Geometry: final body of the model. Coordinates: model frame, mm. A direction names the side the tool comes from. Round coordinates to 2 decimals unless told otherwise and drop trailing zeros. Loops run counter-clockwise (first coordinate to the right, second up) from the corner with the lowest first, then second, coordinate; pieces in that order, holes last. Notation, with made-up numbers: (83.5, 23.25) -> (124.5, 23.25) arc R9 cw to (124.5, 33.25) -> close; hole circle Ø10 at (44, 23). An arc over 180 degrees is marked (long way). Answer in a Markdown table with one row per item.
```python
from build123d import *

# Parameters (mm, degrees)
IZIM1_W                     = 170
IZIM1_H                     = 8
Y_KSEKLIK_EKSTR_ZYON1_DEPTH = 60
IZIM2_R                     = 1.6
IZIM2_R_2                   = 2.1
KES_EKSTR_ZYON1_DEPTH       = 5
IZIM3_R                     = 3.4
KES_EKSTR_ZYON2_DEPTH       = 2.7
IZIM4_R                     = 4.4
KES_EKSTR_ZYON3_DEPTH       = 3.5
RADYUS1_R                   = 4
KES_EKSTR_ZYON4_DEPTH       = 10


with BuildPart() as part:
    # Çizim1 → Yükseklik-Ekstrüzyon1 (new, symmetric)
    with BuildSketch(Plane.XY):
        Rectangle(IZIM1_W, IZIM1_H)
    extrude(amount=Y_KSEKLIK_EKSTR_ZYON1_DEPTH, both=True)

    # Çizim2 → Kes-Ekstrüzyon1 (cut, symmetric)
    with BuildSketch(Plane(origin=(0, 0, 0), x_dir=(1, 0, 0), z_dir=(0, 1, 0))):
        with Locations(Location((0, 56, 0), (0, 0, 270))):
            Circle(IZIM2_R)
        with Locations(Location((0, -56, 0), (0, 0, 270))):
            Circle(IZIM2_R)
        with Locations(Location((-76, 0, 0), (0, 0, 270))):
            Circle(IZIM2_R_2)
        with Locations(Location((76, 0, 0), (0, 0, 270))):
            Circle(IZIM2_R_2)
    extrude(amount=KES_EKSTR_ZYON1_DEPTH, both=True, mode=Mode.SUBTRACT)

    # Çizim3 → Kes-Ekstrüzyon2 (cut)
    with BuildSketch(Plane.XZ.offset(4)):
        with Locations(Location((0, -56, 0), (0, 0, 270))):
            Circle(IZIM3_R)
        with Locations(Location((0, 56, 0), (0, 0, 270))):
            Circle(IZIM3_R)
    extrude(amount=-KES_EKSTR_ZYON2_DEPTH, mode=Mode.SUBTRACT)

    # Çizim4 → Kes-Ekstrüzyon3 (cut)
    with BuildSketch(Plane.XZ.offset(4)):
        with Locations(Location((-76, 0, 0), (0, 0, 270))):
            Circle(IZIM4_R)
        with Locations(Location((76, 0, 0), (0, 0, 270))):
            Circle(IZIM4_R)
    extrude(amount=-KES_EKSTR_ZYON3_DEPTH, mode=Mode.SUBTRACT)

    # Radyus1
    # the kernel refuses this fillet: 4 mm, written as the material it takes off along each edge
    with BuildSketch(Plane(origin=(-95, -4, 60), x_dir=(0, 0, -1), z_dir=(1, 0, 0))) as radyus1_piece_1:
        with BuildLine():
            CenterArc((RADYUS1_R, RADYUS1_R), RADYUS1_R, 180, 90)
            Line((0, RADYUS1_R), (0, 0))
            Line((0, 0), (RADYUS1_R, 0))
        make_face()
    extrude(amount=190, mode=Mode.SUBTRACT)
    with BuildSketch(Plane(origin=(-95, -4, -60), x_dir=(0, 0, 1), z_dir=(1, 0, 0))) as radyus1_piece_2:
        with BuildLine():
            CenterArc((RADYUS1_R, -RADYUS1_R), RADYUS1_R, 90, 90)
            Line((0, -RADYUS1_R), (0, 0))
            Line((0, 0), (RADYUS1_R, 0))
        make_face()
    extrude(amount=190, mode=Mode.SUBTRACT)

    # Çizim6 → Kes-Ekstrüzyon4 (cut, symmetric)
    with BuildSketch(Plane(origin=(0, 0, 0), x_dir=(1, 0, 0), z_dir=(0, 1, 0))):
        with BuildLine():
            Line((4.5, -43.24922609), (58.973465944, -43.24922609))
            ThreePointArc((58.973465944, -43.24922609), (59.680572726, -43.542119309), (59.973465944, -44.24922609))
            Line((59.973465944, -44.24922609), (59.973465944, -45.74922609))
            ThreePointArc((59.973465944, -45.74922609), (59.680572726, -46.456332871), (58.973465944, -46.74922609))
            Line((58.973465944, -46.74922609), (-59.026534056, -46.74922609))
            ThreePointArc((-59.026534056, -46.74922609), (-59.733640837, -46.456332871), (-60.026534056, -45.74922609))
            Line((-60.026534056, -45.74922609), (-60.026534056, -44.24922609))
            ThreePointArc((-60.026534056, -44.24922609), (-59.733640837, -43.542119309), (-59.026534056, -43.24922609))
            Line((-59.026534056, -43.24922609), (-4.5, -43.24922609))
            Line((-4.5, -43.24922609), (4.5, -43.24922609))
        make_face()
        with BuildLine():
            Line((-59.026534056, -1.74922609), (-4.5, -1.74922609))
            Line((-4.5, -1.74922609), (4.5, -1.74922609))
            Line((4.5, -1.74922609), (58.973465944, -1.74922609))
            ThreePointArc((58.973465944, -1.74922609), (59.680572726, -1.456332871), (59.973465944, -0.74922609))
            Line((59.973465944, -0.74922609), (59.973465944, 0.747733475))
            ThreePointArc((59.973465944, 0.747733475), (59.68059176, 1.454821222), (58.973519783, 1.747733474))
            Line((58.973519783, 1.747733474), (4.499892323, 1.750666239))
            Line((4.499892323, 1.750666239), (-4.5, 1.75077391))
            Line((-4.5, 1.75077391), (-59.026534056, 1.75077391))
            ThreePointArc((-59.026534056, 1.75077391), (-59.733640837, 1.457880691), (-60.026534056, 0.75077391))
            Line((-60.026534056, 0.75077391), (-60.026534056, -0.74922609))
            ThreePointArc((-60.026534056, -0.74922609), (-59.733640837, -1.456332871), (-59.026534056, -1.74922609))
        make_face()
        with BuildLine():
            Line((4.5, -28.24922609), (58.973465944, -28.24922609))
            ThreePointArc((58.973465944, -28.24922609), (59.680572726, -28.542119309), (59.973465944, -29.24922609))
            Line((59.973465944, -29.24922609), (59.973465944, -30.74922609))
            ThreePointArc((59.973465944, -30.74922609), (59.680572726, -31.456332871), (58.973465944, -31.74922609))
            Line((58.973465944, -31.74922609), (4.5, -31.74922609))
            Line((4.5, -31.74922609), (-4.5, -31.74922609))
            Line((-4.5, -31.74922609), (-59.026534056, -31.74922609))
            ThreePointArc((-59.026534056, -31.74922609), (-59.733640837, -31.456332871), (-60.026534056, -30.74922609))
            Line((-60.026534056, -30.74922609), (-60.026534056, -29.24922609))
            ThreePointArc((-60.026534056, -29.24922609), (-59.733640837, -28.542119309), (-59.026534056, -28.24922609))
            Line((-59.026534056, -28.24922609), (-4.5, -28.24922609))
            Line((-4.5, -28.24922609), (4.5, -28.24922609))
        make_face()
        with BuildLine():
            Line((-60.026534056, 14.25077391), (-60.026534056, 15.75077391))
            ThreePointArc((-60.026534056, 15.75077391), (-59.733640837, 16.457880691), (-59.026534056, 16.75077391))
            Line((-59.026534056, 16.75077391), (-4.5, 16.75077391))
            Line((-4.5, 16.75077391), (4.5, 16.75077391))
            Line((4.5, 16.75077391), (58.973465944, 16.75077391))
            ThreePointArc((58.973465944, 16.75077391), (59.680572726, 16.457880691), (59.973465944, 15.75077391))
            Line((59.973465944, 15.75077391), (59.973465944, 14.25077391))
            ThreePointArc((59.973465944, 14.25077391), (59.680572726, 13.543667129), (58.973465944, 13.25077391))
            Line((58.973465944, 13.25077391), (4.5, 13.25077391))
            Line((4.5, 13.25077391), (-4.5, 13.25077391))
            Line((-4.5, 13.25077391), (-59.026534056, 13.25077391))
            ThreePointArc((-59.026534056, 13.25077391), (-59.733640837, 13.543667129), (-60.026534056, 14.25077391))
        make_face()
        with BuildLine():
            Line((-60.026534056, 29.25077391), (-60.026534056, 30.75077391))
            ThreePointArc((-60.026534056, 30.75077391), (-59.733640837, 31.457880691), (-59.026534056, 31.75077391))
            Line((-59.026534056, 31.75077391), (-4.5, 31.75077391))
            Line((-4.5, 31.75077391), (4.5, 31.75077391))
            Line((4.5, 31.75077391), (58.973465944, 31.75077391))
            ThreePointArc((58.973465944, 31.75077391), (59.680572726, 31.457880691), (59.973465944, 30.75077391))
            Line((59.973465944, 30.75077391), (59.973465944, 29.25077391))
            ThreePointArc((59.973465944, 29.25077391), (59.680572726, 28.543667129), (58.973465944, 28.25077391))
            Line((58.973465944, 28.25077391), (4.5, 28.25077391))
            Line((4.5, 28.25077391), (-4.5, 28.25077391))
            Line((-4.5, 28.25077391), (-59.026534056, 28.25077391))
            ThreePointArc((-59.026534056, 28.25077391), (-59.733640837, 28.543667129), (-60.026534056, 29.25077391))
        make_face()
        with BuildLine():
            Line((-60.026534056, 44.25077391), (-60.026534056, 45.75077391))
            ThreePointArc((-60.026534056, 45.75077391), (-59.733640837, 46.457880691), (-59.026534056, 46.75077391))
            Line((-59.026534056, 46.75077391), (58.973465944, 46.75077391))
            ThreePointArc((58.973465944, 46.75077391), (59.680572726, 46.457880691), (59.973465944, 45.75077391))
            Line((59.973465944, 45.75077391), (59.973465944, 44.25077391))
            ThreePointArc((59.973465944, 44.25077391), (59.680572726, 43.543667129), (58.973465944, 43.25077391))
            Line((58.973465944, 43.25077391), (4.5, 43.25077391))
            Line((4.5, 43.25077391), (-4.5, 43.25077391))
            Line((-4.5, 43.25077391), (-59.026534056, 43.25077391))
            ThreePointArc((-59.026534056, 43.25077391), (-59.733640837, 43.543667129), (-60.026534056, 44.25077391))
        make_face()
        with BuildLine():
            Line((-60.026534056, -15.74922609), (-60.026534056, -14.24922609))
            ThreePointArc((-60.026534056, -14.24922609), (-59.733640837, -13.542119309), (-59.026534056, -13.24922609))
            Line((-59.026534056, -13.24922609), (-4.5, -13.24922609))
            Line((-4.5, -13.24922609), (4.5, -13.24922609))
            Line((4.5, -13.24922609), (58.973465944, -13.24922609))
            ThreePointArc((58.973465944, -13.24922609), (59.680572726, -13.542119309), (59.973465944, -14.24922609))
            Line((59.973465944, -14.24922609), (59.973465944, -15.74922609))
            ThreePointArc((59.973465944, -15.74922609), (59.680572726, -16.456332871), (58.973465944, -16.74922609))
            Line((58.973465944, -16.74922609), (4.5, -16.74922609))
            Line((4.5, -16.74922609), (-4.5, -16.74922609))
            Line((-4.5, -16.74922609), (-59.026534056, -16.74922609))
            ThreePointArc((-59.026534056, -16.74922609), (-59.733640837, -16.456332871), (-60.026534056, -15.74922609))
        make_face()
    extrude(amount=KES_EKSTR_ZYON4_DEPTH, both=True, mode=Mode.SUBTRACT)


solid = part.part
```
Item 1: Set-up query: faces 1 (the cylindrical face through (-80.295, -2.274, 0.954)), 2 (the flat face through (-1, 0, -16.751)), 3 (the flat face through (-1, 4, -12)). Return all of +Z, -Z, +X, -X, +Y, -Y with unobstructed straight access to the full face (end or side cutting, diameter ignored); none if empty.
Ans:
| item | result |
|---|---|
| face 1 | -Y |
| face 2 | +Y, -Y |
| face 3 | +Z, -Z, +X, -X, +Y |
Item 2: Ray query, L1, parallel to X at y = -1.35, z = 0; L2, parallel to X at y = 1.6, z = 0; L3, parallel to X at y = -3, z = 15.5. Return the intervals inside material, ascending.
Ans:
| item | result |
|---|---|
| L1 | -85 to -80.4, -71.6 to -60.03, 59.97 to 71.6, 80.4 to 85 |
| L2 | -85 to -78.1, -73.9 to -60.03, 59.97 to 73.9, 78.1 to 85 |
| L3 | -85 to -60.03, 59.97 to 85 |
Item 3: Mould query, pull axis X, two halves, no side actions, for faces 4 (the flat face through (1, 0, 16.749)), 5 (the flat face through (-1, 2, 60)), 6 (the flat face through (85, 0, 1)). Classes: released by +X, released by -X, zero draft, split by the parting line, or undercut.
Ans:
| item | result |
|---|---|
| face 4 | undercut |
| face 5 | zero draft |
| face 6 | released by +X |
Item 4: Section query A-A, the plane x = -76. Output: boundary loops of the cut face in (y, z), and give its area (3 significant figures).
Ans:
| item | result |
|---|---|
| outline | (-4, -56) arc R4 ccw to (0, -60) -> (4, -60) -> (4, -2.1) -> (-0.5, -2.1) -> (-0.5, -4.4) -> (-4, -4.4) -> close; (-4, 4.4) -> (-0.5, 4.4) -> (-0.5, 2.1) -> (4, 2.1) -> (4, 60) -> (0, 60) arc R4 ccw to (-4, 56) -> close |
| area | 903 mm2 |
Item 5: Section query B-B, the plane x = -33. State how many separate pieces and enclosed holes the cut face has, and give its area (3 significant figures).
Ans:
| item | result |
|---|---|
| separate pieces | 8 |
| enclosed holes | 0 |
| area | 757 mm2 |
Item 6: First-contact query: P1, Ø5.5, axis at x = 76, z = 0, coming from the -Y side; P2, Ø2.5, axis at x = 0.5, y = -1.5, coming from the +Z side; P3, Ø2, axis at x = -1.5, z = 54.5, coming from the -Y side. Flat tips, straight axial feed; report the tip coordinate or a pass-through.
Ans:
| item | result |
|---|---|
| P1 | y = -0.5 |
| P2 | z = 59.99 |
| P3 | y = -1.3 |
